from build123d import *

# Parameters (mm, degrees)
SKETCH2_R      = 0.9906
EXTRUDE1_DEPTH = 1.27
FILLET1_R      = 0.254


with BuildPart() as part:
    # Sketch2 → Extrude1 (new body)
    with BuildSketch(Plane(origin=(0, 0, 0), x_dir=(1, 0, 0), z_dir=(0, 1, 0))):
        with BuildLine():
            Line((6.703697653, -14.37612601), (5.655670247, -12.128623984))
            ThreePointArc((5.655670247, -12.128623984), (5.854908275, -9.851322904), (7.926727876, -8.885217558))
            Line((7.926727876, -8.885217558), (11.125604013, -9.165082956))
            ThreePointArc((11.125604013, -9.165082956), (0, 12.9159), (-11.125604013, -9.165082956))
            Line((-11.125604013, -9.165082956), (-7.926727876, -8.885217558))
            ThreePointArc((-7.926727876, -8.885217558), (-5.854908275, -9.851322904), (-5.655670247, -12.128623984))
            Line((-5.655670247, -12.128623984), (-6.703697653, -14.37612601))
            ThreePointArc((-6.703697653, -14.37612601), (0, 15.8623), (6.703697653, -14.37612601))
        make_face()
        with Locations((7.727489848, -11.162518638)):
            Circle(SKETCH2_R, mode=Mode.SUBTRACT)
        with Locations((-7.727489848, -11.162518638)):
            Circle(SKETCH2_R, mode=Mode.SUBTRACT)
    extrude(amount=-EXTRUDE1_DEPTH)

    # Fillet1
    fillet1_edges = [part.edges().sort_by_distance(p)[0] for p in [
        (11.125604013, -0.635, 9.165082956),
        (-11.125604013, -0.635, 9.165082956),
    ]]
    fillet(fillet1_edges, radius=FILLET1_R)


solid = part.part
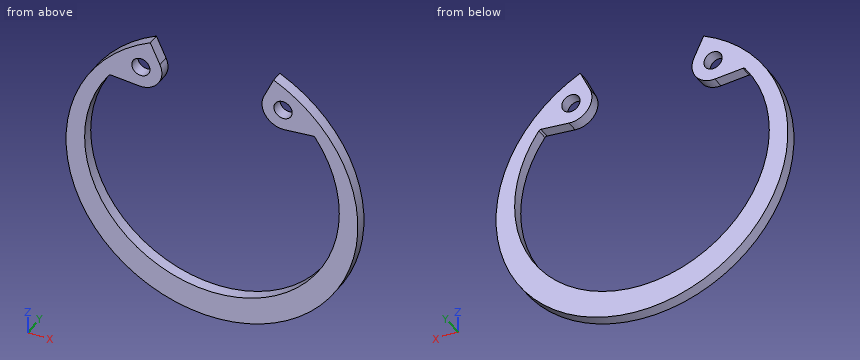
Work out the finished part from the listing and answer in its coordinate system (mm). Give positions to 0.01 mm unless a question says otherwise; leave off trailing zeros. Loops run counter-clockwise (first coordinate to the right, second up) from the corner with the lowest first, then second, coordinate; pieces in that order, holes last. Notation, with made-up numbers: (-26.5, 35) -> (-6.5, 35) arc R22 cw to (-6.5, 63) -> close; hole circle Ø10 at (-29.5, 3). An arc over 180 degrees is marked (long way). Use a Markdown table: item, result. Add a question column.
1. Section D-D on x = 0 is taken. Determine the outline of the cut face in (y, z).
2. Find the intervals of material crossed by probe 1 along X at (y, z) = (-0.6, 0.5); probe 2 along Z at (x, y) = (7, -0.35); probe 3 along Z at (x, y) = (-8.5, -1), in increasing order.
3. Section B-B on z = -6 is taken. Determine the outline of the cut face in (x, y).
4. Section C-C on y = -0.8 is taken. Determine the outline of the cut face in (x, z).
5. Section A-A on x = 10 is taken. Determine the outline of the cut face in (y, z).
Results below:
| question | item | result |
|---|---|---|
| 1 | outline | (-1.27, -15.86) -> (0, -15.86) -> (0, -12.92) -> (-1.27, -12.92) -> close |
| 2 | probe 1 | x = -15.85 to -13.84, 13.84 to 15.85 |
| 2 | probe 2 | z = -14.23 to -11.02, 9 to 10.49, 11.83 to 14.23 |
| 2 | probe 3 | z = -13.39 to -10, 8.94 to 10.54, 11.78 to 13.39 |
| 3 | outline | (-14.68, -1.27) -> (-11.99, -1.27) -> (-11.99, 0) -> (-14.68, 0) -> close; (11.99, -1.27) -> (14.68, -1.27) -> (14.68, 0) -> (11.99, 0) -> close |
| 4 | outline | (-11.21, 9.05) arc R0.25 cw to (-10.98, 9.15) -> (-7.93, 8.89) arc R2.29 ccw to (-5.66, 12.13) -> (-6.7, 14.38) arc R15.86 ccw (long way) to (6.7, 14.38) -> (5.66, 12.13) arc R2.29 ccw to (7.93, 8.89) -> (10.98, 9.15) arc R0.25 cw to (11.21, 9.05) arc R13.84 cw (long way) to start; hole circle Ø1.98 at (-7.73, 11.16); hole circle Ø1.98 at (7.73, 11.16) |
| 5 | outline | (-1.27, -12.31) -> (0, -12.31) -> (0, -8.65) -> (-1.27, -8.65) -> close; (-1.27, 9.07) -> (0, 9.07) -> (0, 12.31) -> (-1.27, 12.31) -> close |
